```python
from build123d import *

# Parameters (mm, degrees)
SKETCH1_R           = 6.604
BOSS_EXTRUDE3_DEPTH = 152.4


with BuildPart() as part:
    # Sketch1 → Boss-Extrude3 (new body)
    with BuildSketch(Plane(origin=(0, 0, 0), x_dir=(1, 0, 0), z_dir=(0, 1, 0))):
        with BuildLine():
            Line((-1.761094277, -12.824695235), (-0.744188415, -14.586027856))
            ThreePointArc((-0.744188415, -14.586027856), (0, -14.605), (0.744188415, -14.586027856))
            Line((0.744188415, -14.586027856), (1.761094277, -12.824695235))
            ThreePointArc((1.761094277, -12.824695235), (1.86082516, -12.676971002), (1.980255064, -12.544663801))
            ThreePointArc((1.980255064, -12.544663801), (2.640478473, -12.422474529), (3.293321424, -12.26556293))
            ThreePointArc((3.293321424, -12.26556293), (3.456240258, -12.337855055), (3.607433811, -12.432243652))
            Line((3.607433811, -12.432243652), (5.25282206, -13.62768819))
            ThreePointArc((5.25282206, -13.62768819), (5.940388672, -13.342331409), (6.612521952, -13.022310795))
            Line((6.612521952, -13.022310795), (6.825113166, -10.999640503))
            ThreePointArc((6.825113166, -10.999640503), (6.856137002, -10.824123497), (6.911427462, -10.654678336))
            ThreePointArc((6.911427462, -10.654678336), (7.464872704, -10.274515829), (7.997452719, -9.8656348))
            ThreePointArc((7.997452719, -9.8656348), (8.175690336, -9.865411882), (8.35220382, -9.890144198))
            Line((8.35220382, -9.890144198), (10.34157188, -10.312997433))
            ThreePointArc((10.34157188, -10.312997433), (10.853630176, -9.772652506), (11.33749037, -9.206917894))
            Line((11.33749037, -9.206917894), (10.709007984, -7.272647999))
            ThreePointArc((10.709007984, -7.272647999), (10.66596047, -7.099686705), (10.647551263, -6.922402191))
            ThreePointArc((10.647551263, -6.922402191), (10.998522628, -6.35), (11.318751785, -5.759848786))
            ThreePointArc((11.318751785, -5.759848786), (11.481489281, -5.687149371), (11.652801912, -5.637948964))
            Line((11.652801912, -5.637948964), (13.642169972, -5.215095729))
            ThreePointArc((13.642169972, -5.215095729), (13.89018042, -4.513193203), (14.102103706, -3.799565247))
            Line((14.102103706, -3.799565247), (12.741218033, -2.288148587))
            ThreePointArc((12.741218033, -2.288148587), (12.631542476, -2.147649583), (12.542616721, -1.99317982))
            ThreePointArc((12.542616721, -1.99317982), (12.630428071, -1.327511483), (12.682935839, -0.658132591))
            ThreePointArc((12.682935839, -0.658132591), (12.802034423, -0.525527067), (12.938524691, -0.410901134))
            Line((12.938524691, -0.410901134), (14.58391294, 0.784543404))
            ThreePointArc((14.58391294, 0.784543404), (14.524992282, 1.526638206), (14.428335197, 2.264766749))
            Line((14.428335197, 2.264766749), (12.570355734, 3.091992503))
            ThreePointArc((12.570355734, 3.091992503), (12.413016034, 3.175735662), (12.268949801, 3.280681449))
            ThreePointArc((12.268949801, 3.280681449), (12.078417757, 3.924515829), (11.854125066, 4.557380709))
            ThreePointArc((11.854125066, 4.557380709), (11.908991511, 4.726963641), (11.987059008, 4.887195235))
            Line((11.987059008, 4.887195235), (13.003964871, 6.648527856))
            ThreePointArc((13.003964871, 6.648527856), (12.648301022, 7.3025), (12.259776456, 7.9375))
            Line((12.259776456, 7.9375), (10.22596473, 7.9375))
            ThreePointArc((10.22596473, 7.9375), (10.048166351, 7.950007361), (9.873870001, 7.987283092))
            ThreePointArc((9.873870001, 7.987283092), (9.437939284, 8.497958701), (8.975628378, 8.984881481))
            ThreePointArc((8.975628378, 8.984881481), (8.956775776, 9.162119392), (8.962921923, 9.340251148))
            Line((8.962921923, 9.340251148), (9.175513137, 11.362921441))
            ThreePointArc((9.175513137, 11.362921441), (8.58460361, 11.815693203), (7.971390989, 12.237767391))
            Line((7.971390989, 12.237767391), (6.113411525, 11.410541637))
            ThreePointArc((6.113411525, 11.410541637), (5.945897421, 11.349650564), (5.771508377, 11.312810926))
            ThreePointArc((5.771508377, 11.312810926), (5.165555367, 11.602027312), (4.545164002, 11.85881462))
            ThreePointArc((4.545164002, 11.85881462), (4.455852141, 12.013061465), (4.389014213, 12.178292785))
            Line((4.389014213, 12.178292785), (3.760531826, 14.11256268))
            ThreePointArc((3.760531826, 14.11256268), (3.036550244, 14.285845709), (2.304679602, 14.422013623))
            Line((2.304679602, 14.422013623), (0.943793928, 12.910596963))
            ThreePointArc((0.943793928, 12.910596963), (0.81552881, 12.786836076), (0.671200521, 12.682250978))
            ThreePointArc((0.671200521, 12.682250978), (0, 12.7), (-0.671200521, 12.682250978))
            ThreePointArc((-0.671200521, 12.682250978), (-0.81552881, 12.786836076), (-0.943793928, 12.910596963))
            Line((-0.943793928, 12.910596963), (-2.304679602, 14.422013623))
            ThreePointArc((-2.304679602, 14.422013623), (-3.036550244, 14.285845709), (-3.760531826, 14.11256268))
            Line((-3.760531826, 14.11256268), (-4.389014213, 12.178292785))
            ThreePointArc((-4.389014213, 12.178292785), (-4.455852141, 12.013061465), (-4.545164002, 11.85881462))
            ThreePointArc((-4.545164002, 11.85881462), (-5.165555367, 11.602027312), (-5.771508377, 11.312810926))
            ThreePointArc((-5.771508377, 11.312810926), (-5.945897421, 11.349650564), (-6.113411525, 11.410541637))
            Line((-6.113411525, 11.410541637), (-7.971390989, 12.237767391))
            ThreePointArc((-7.971390989, 12.237767391), (-8.58460361, 11.815693203), (-9.175513137, 11.362921441))
            Line((-9.175513137, 11.362921441), (-8.962921923, 9.340251148))
            ThreePointArc((-8.962921923, 9.340251148), (-8.956775776, 9.162119392), (-8.975628378, 8.984881481))
            ThreePointArc((-8.975628378, 8.984881481), (-9.437939284, 8.497958701), (-9.873870001, 7.987283092))
            ThreePointArc((-9.873870001, 7.987283092), (-10.048166351, 7.950007361), (-10.22596473, 7.9375))
            Line((-10.22596473, 7.9375), (-12.259776456, 7.9375))
            ThreePointArc((-12.259776456, 7.9375), (-12.648301022, 7.3025), (-13.003964871, 6.648527856))
            Line((-13.003964871, 6.648527856), (-11.987059008, 4.887195235))
            ThreePointArc((-11.987059008, 4.887195235), (-11.908991511, 4.726963641), (-11.854125066, 4.557380709))
            ThreePointArc((-11.854125066, 4.557380709), (-12.078417757, 3.924515829), (-12.268949801, 3.280681449))
            ThreePointArc((-12.268949801, 3.280681449), (-12.413016034, 3.175735662), (-12.570355734, 3.091992503))
            Line((-12.570355734, 3.091992503), (-14.428335197, 2.264766749))
            ThreePointArc((-14.428335197, 2.264766749), (-14.524992282, 1.526638206), (-14.58391294, 0.784543404))
            Line((-14.58391294, 0.784543404), (-12.938524691, -0.410901134))
            ThreePointArc((-12.938524691, -0.410901134), (-12.802034423, -0.525527067), (-12.682935839, -0.658132591))
            ThreePointArc((-12.682935839, -0.658132591), (-12.630428071, -1.327511483), (-12.542616721, -1.99317982))
            ThreePointArc((-12.542616721, -1.99317982), (-12.631542476, -2.147649583), (-12.741218033, -2.288148587))
            Line((-12.741218033, -2.288148587), (-14.102103706, -3.799565247))
            ThreePointArc((-14.102103706, -3.799565247), (-13.89018042, -4.513193203), (-13.642169972, -5.215095729))
            Line((-13.642169972, -5.215095729), (-11.652801912, -5.637948964))
            ThreePointArc((-11.652801912, -5.637948964), (-11.481489281, -5.687149371), (-11.318751785, -5.759848786))
            ThreePointArc((-11.318751785, -5.759848786), (-10.998522628, -6.35), (-10.647551263, -6.922402191))
            ThreePointArc((-10.647551263, -6.922402191), (-10.66596047, -7.099686705), (-10.709007984, -7.272647999))
            Line((-10.709007984, -7.272647999), (-11.33749037, -9.206917894))
            ThreePointArc((-11.33749037, -9.206917894), (-10.853630176, -9.772652506), (-10.34157188, -10.312997433))
            Line((-10.34157188, -10.312997433), (-8.35220382, -9.890144198))
            ThreePointArc((-8.35220382, -9.890144198), (-8.175690336, -9.865411882), (-7.997452719, -9.8656348))
            ThreePointArc((-7.997452719, -9.8656348), (-7.464872704, -10.274515829), (-6.911427462, -10.654678336))
            ThreePointArc((-6.911427462, -10.654678336), (-6.856137002, -10.824123497), (-6.825113166, -10.999640503))
            Line((-6.825113166, -10.999640503), (-6.612521952, -13.022310795))
            ThreePointArc((-6.612521952, -13.022310795), (-5.940388672, -13.342331409), (-5.25282206, -13.62768819))
            Line((-5.25282206, -13.62768819), (-3.607433811, -12.432243652))
            ThreePointArc((-3.607433811, -12.432243652), (-3.456240258, -12.337855055), (-3.293321424, -12.26556293))
            ThreePointArc((-3.293321424, -12.26556293), (-2.640478473, -12.422474529), (-1.980255064, -12.544663801))
            ThreePointArc((-1.980255064, -12.544663801), (-1.86082516, -12.676971002), (-1.761094277, -12.824695235))
        make_face()
        with Locations(Location((0, 0, 0), (0, 0, 90))):
            Circle(SKETCH1_R, mode=Mode.SUBTRACT)
    extrude(amount=BOSS_EXTRUDE3_DEPTH)


solid = part.part
```
Can you work these out from the model? Positions are in its coordinate system, mm. Round coordinates to 2 decimals unless told otherwise and drop trailing zeros.
Item 1: If we mould it in two halves opening along Z, with no side actions, what happens to faces 1 (the cylindrical face through (-1.98, 75.13, -6.3)), 2 (the flat face through (3, 152.4, 6.3))? For each: +Z half, -Z half, draft (parallel to the pull), parting line (faces both ways), or undercut.
Item 2: Will these pins go through, and if not, where does the flat tip stop? pin 1 Ø2 at (x, z) = (11, 10) entering from +Y; pin 2 Ø3 at (x, y) = (-11, 33) entering from +Z; pin 3 Ø8 at (x, y) = (10.5, 103) entering from -Z; pin 4 Ø0.6 at (x, y) = (-11, 91.5) entering from -Z.
Item 3: Please list where these lines run through material, in increasing order: L1, parallel to X at y = 131, z = -11.5; L2, parallel to X at y = 52, z = -0.5; L3, parallel to Z at x = -0.5, y = 94.
Reported:
1. face 1: undercut
1. face 2: draft
2. pin 1: stops at y = 152.4
2. pin 2: stops at z = 10.31
2. pin 3: stops at z = -12.24
2. pin 4: stops at z = -7.94
3. L1: x = -9 to -6.31, -5.39 to 5.39, 6.31 to 9
3. L2: x = -14.19 to -6.59, 6.59 to 14.19
3. L3: z = -12.69 to -6.59, 6.59 to 14.6
